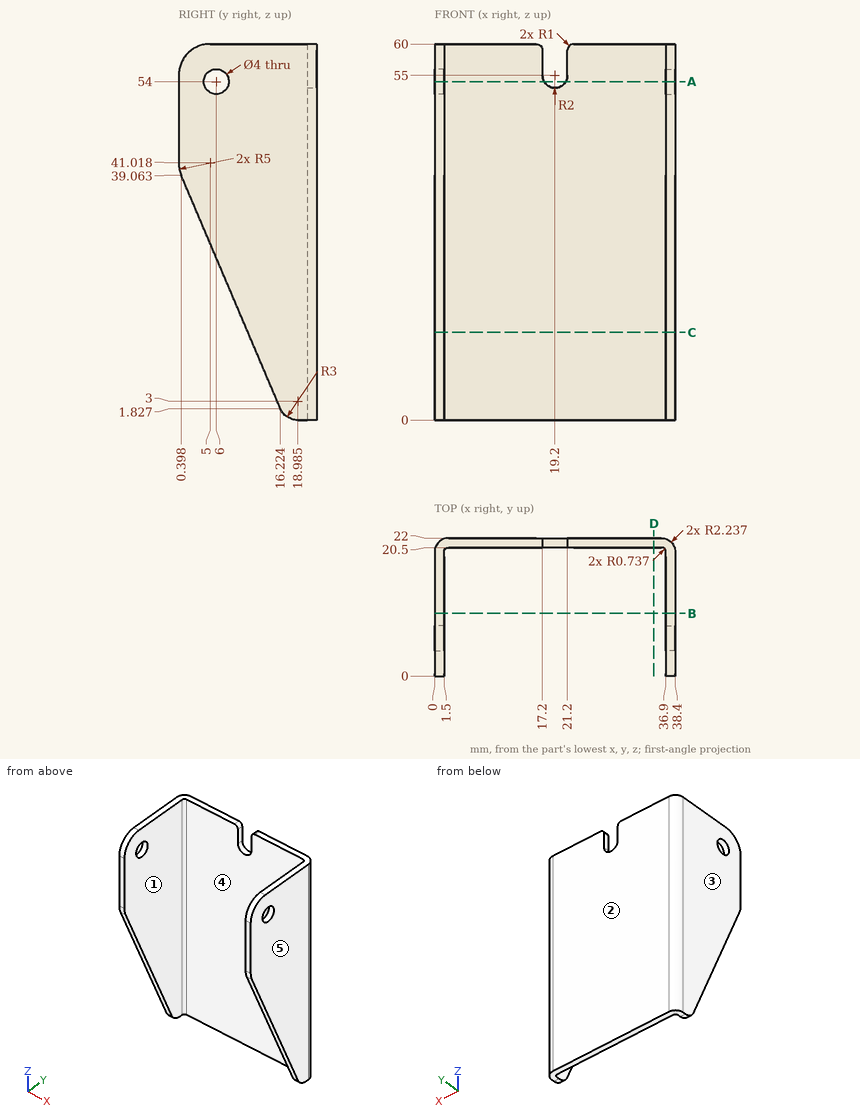
Here's the drawing with two shaded views (mm, measured from the low corner). I have some questions. A direction names the side the tool comes from. Round coordinates to 2 decimals unless told otherwise and drop trailing zeros. Loops run counter-clockwise (first coordinate to the right, second up) from the corner with the lowest first, then second, coordinate; pieces in that order, holes last.
1. Suppose I cut it at C-C, the plane z = 14. Please give me the cut outline in (x, y).
Answers:
outline: (0, 11.05) - (1.5, 11.05) - (1.5, 19.76) arc R0.74 cw to (2.24, 20.5) - (36.16, 20.5) arc R0.74 cw to (36.9, 19.76) - (36.9, 11.05) - (38.4, 11.05) - (38.4, 19.76) arc R2.24 ccw to (36.16, 22) - (2.24, 22) arc R2.24 ccw to (0, 19.76) - close
2. Suppose I cut it at A-A, the plane z = 54. Please give me the cut outline in (x, y).
Answers:
outline: (0, 0) - (1.5, 0) - (1.5, 4) - (0, 4) - close; (0, 8) - (1.5, 8) - (1.5, 19.76) arc R0.74 cw to (2.24, 20.5) - (17.47, 20.5) - (17.47, 22) - (2.24, 22) arc R2.24 ccw to (0, 19.76) - close; (20.93, 20.5) - (36.16, 20.5) arc R0.74 cw to (36.9, 19.76) - (36.9, 8) - (38.4, 8) - (38.4, 19.76) arc R2.24 ccw to (36.16, 22) - (20.93, 22) - close; (36.9, 0) - (38.4, 0) - (38.4, 4) - (36.9, 4) - close
3. For the marked faces 1 and 2, which set-ups out of +Z, -Z, +X, -X, +Y, -Y let a thin tool reach every point of the face, with its end or its side?
Answers:
face 1: +Z, -Z, -Y
face 2: +Z, -Z, +X, -X, +Y
4. Will these pins go through, and if not, where does the flat tip stop? pin 1 (8 mm diameter, centred on y = 17, z = 53, fed in from -X); pin 2 (1.6 mm diameter, centred on y = 21.5, z = 57, fed in from -X) (1 decimal); pin 3 (17 mm diameter, centred on x = 19.5, z = 32.5, fed in from -Y); pin 4 (2.5 mm diameter, centred on y = 6, z = 54, fed in from +X).
Answers:
pin 1: stops at x = 0
pin 2: stops at x = 0.2
pin 3: stops at y = 20.5
pin 4: passes through
5. Thinking about a two-plate mould opening in X: for the marked faces 3, 4 and 5, which applies, released by +X, released by -X, zero draft, split by the parting line, or undercut?
Answers:
face 3: released by -X
face 4: undercut
face 5: released by +X
6. Suppose I cut it at B-B, the plane y = 10. Please give me the cut outline in (x, z).
Answers:
outline: (0, 16.47) - (1.5, 16.47) - (1.5, 60) - (0, 60) - close; (36.9, 16.47) - (38.4, 16.47) - (38.4, 60) - (36.9, 60) - close
7. If I drill on probe 1 along X at (y, z) = (18.75, 48); probe 2 along Y at (x, z) = (3, 48); probe 3 along X at (y, z) = (21.25, 15) (1 decimal), over which ranges is the centre line in solid material (lowest first)?
Answers:
probe 1: x = 0 to 1.5, 36.9 to 38.4
probe 2: y = 20.5 to 22
probe 3: x = 0.6 to 37.8
8. Suppose I cut it at D-D, the plane x = 35. Please give me the cut outline in (y, z).
Answers:
outline: (20.5, 0) - (22, 0) - (22, 60) - (20.5, 60) - close
